Autodesk Inventor part; units mm, degrees
ref_plane "YZ Plane" through (0, 0, 0) normal (1, 0, 0) x (0, 1, 0)
ref_plane "XZ Plane" through (0, 0, 0) normal (0, 1, 0) x (-1, 0, 0)
ref_plane "XY Plane" through (0, 0, 0) normal (0, 0, 1) x (1, 0, 0)
sketch "Boceto1" plane through (0, 0, 0) normal (0, 1, 0) x (-1, 0, 0)
  line L0 (-11.1918, 40) -> (11.1918, 40)
  line L1 (11.1918, 40) -> (11.1918, -40)
  line L2 (11.1918, -40) -> (-11.1918, -40)
  line L3 (-11.1918, -40) -> (-11.1918, 40)
  line L4 (-11.1918, 40) -> (11.1918, -40) construction
  line L5 (11.1918, 40) -> (-11.1918, -40) construction
  circle A0 centre (0, 30) radius 2.7
  circle A1 centre (0, -30) radius 2.7
  point P0 (0, 0)
  dimension "d0" = 5.4
  dimension "d1" = 80
  dimension "d2" = 10
  dimension "d3" = 10
extrude "Extrusión1" add sketch "Boceto1" along normal blind 70
sketch "Boceto2" plane through (-11.1918, 0, -40) normal (-1, 0, 0) x (0, 0, 1)
  line L0 (67.5, -15) -> (12.5, -15)
  line L1 (12.5, -15) -> (12.5, 15)
  line L2 (12.5, 15) -> (67.5, 15)
  line L3 (67.5, 15) -> (67.5, -15)
  line L4 (67.5, -15) -> (12.5, 15) construction
  line L5 (12.5, -15) -> (67.5, 15) construction
  point P0 (40, 0)
  dimension "d6" = 55
  dimension "d7" = 30
extrude "Extrusión2" cut sketch "Boceto2" against normal through all
properties part number "LowerJawSupport"
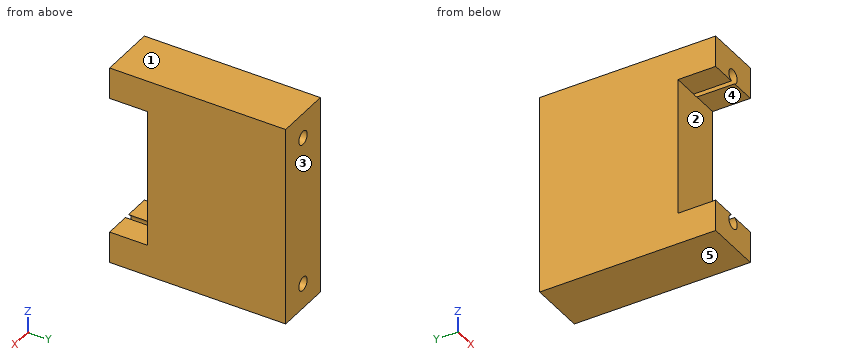
Work out the finished part from the listing and answer in its coordinate system (mm). Face numbers are marked on the shaded views. A direction names the side the tool comes from. Give positions to 0.01 mm unless a question says otherwise; leave off trailing zeros. Loops run counter-clockwise (first coordinate to the right, second up) from the corner with the lowest first, then second, coordinate; pieces in that order, holes last. Notation, with made-up numbers: (38, 3) -> (50, 3) arc R31 cw to (50, 28) -> close; hole circle Ø1 at (6, 42.5). An arc over 180 degrees is marked (long way). Write item = value, one per line. Start each with the question number.
(1) Which of the six approach directions +Z, -Z, +X, -X, +Y, -Y give full straight-line access (tool end or side, diameter ignored) to the marked faces 4 and 5?
(2) Find section C-C on z = -30. Give the vertices of the cut face in (x, y).
(3) Given pin 1 Ø7 at (x, z) = (0, -30) entering from -Y; pin 2 Ø6.5 at (x, z) = (2.5, 5.5) entering from -Y, each flat-ended and moving along its own axis, determine where each tip first touches the part or whether it passes through.
(4) Find the intervals of material crossed by probe 1 along Z at (x, y) = (0, 34.5); probe 2 along X at (y, z) = (17.5, -30); probe 3 along Z at (x, y) = (1, 37), in increasing order. Write a range as from..to.
(5) Find section D-D on z = 26. Give the vertices of the cut face in (x, y), and give its area (3 significant figures).
(6) The mould has two halves that part along Z. Classify the marked faces 1, 2 and 3: +Z half, -Z half, draft (parallel to the pull), parting line (faces both ways), or undercut.
(7) Find section A-A on y = 31. Give the vertices of the cut face in (x, z).
(8) Find section B-B on x = 0. Give the vertices of the cut face in (y, z).
From the geometry:
q1.face_4 = +X, -X, -Y
q1.face_5 = -Z, +X, -X, +Y, -Y
q2.outline = (-11.19, 0) -> (-2.7, 0) -> (-2.7, 70) -> (-11.19, 70) -> close; (2.7, 0) -> (11.19, 0) -> (11.19, 70) -> (2.7, 70) -> close
q3.pin_1 = 0
q3.pin_2 = 15
q4.probe_1 = -40..-32.7, -27.3..27.3, 32.7..40
q4.probe_2 = -11.19..-2.7, 2.7..11.19
q4.probe_3 = -40..-32.51, -27.49..27.49, 32.51..40
q5.outline = (-11.19, 15) -> (11.19, 15) -> (11.19, 70) -> (-11.19, 70) -> close
q5.area = 1,230 mm^2
q6.face_1 = +Z half
q6.face_2 = undercut
q6.face_3 = draft
q7.outline = (-11.19, -40) -> (11.19, -40) -> (11.19, 40) -> (-11.19, 40) -> close; hole circle Ø5.4 at (0, -30); hole circle Ø5.4 at (0, 30)
q8.outline = (0, -40) -> (70, -40) -> (70, -32.7) -> (0, -32.7) -> close; (0, 32.7) -> (70, 32.7) -> (70, 40) -> (0, 40) -> close; (15, -27.3) -> (70, -27.3) -> (70, 27.3) -> (15, 27.3) -> close
